Work out the finished part from the listing and answer in its coordinate system (mm). Round coordinates to 2 decimals unless told otherwise and drop trailing zeros. Order: outer loops, then holes, each group sorted by start corner. A loop starts at its lowest first (then second) coordinate and runs counter-clockwise, first axis right, second up. Notation, with made-up numbers: M -34,73.25 L -23,73.25 A11 ccw -23,93.25 Z; hole C 27,89.25 d5. An arc over 180 degrees is marked long. Answer as a JSON object with one key per item and string values. Group by question number.
from build123d import *

# Parameters (mm, degrees)
BOSS_EXTRUDE1_DEPTH = 13.7
SKETCH3_W           = 0.178571672
SKETCH3_H           = 6.380917094
CUT_EXTRUDE1_DEPTH  = 0.2
SKETCH4_R           = 0.85
BOSS_EXTRUDE3_DEPTH = 7.4
SKETCH5_W           = 0.138137893
SKETCH5_H           = 1.329179466
BOSS_EXTRUDE4_DEPTH = 2.8
SKETCH6_R           = 0.20198457
CUT_EXTRUDE2_DEPTH  = 9.6
REDONDEO1_R         = 0.5


with BuildPart() as part:
    # Sketch1 → Boss-Extrude1 (new body)
    with BuildSketch(Plane.XY):
        with BuildLine():
            Line((-3.31662479, -5), (3.31662479, -5))
            ThreePointArc((3.31662479, -5), (6, 0), (3.31662479, 5))
            Line((3.31662479, 5), (-3.31662479, 5))
            ThreePointArc((-3.31662479, 5), (-6, 0), (-3.31662479, -5))
        make_face()
    extrude(amount=BOSS_EXTRUDE1_DEPTH)

    # Sketch3 → Cut-Extrude1 (cut)
    with BuildSketch(Plane(origin=(0, 5, 0), x_dir=(1, 0, 0), z_dir=(0, 1, 0))):
        with Locations((-2.495957535, -5.684471075)):
            Rectangle(SKETCH3_W, SKETCH3_H)
        with Locations((2.495957535, -5.684471075)):
            Rectangle(SKETCH3_W, SKETCH3_H)
    extrude(amount=-CUT_EXTRUDE1_DEPTH, mode=Mode.SUBTRACT)

    # Sketch4 → Boss-Extrude3 (add)
    with BuildSketch(Plane(origin=(0, 0, 0), x_dir=(-1, 0, 0), z_dir=(0, 0, -1))):
        with Locations(Location((0, 0, 0), (0, 0, 180))):
            Circle(SKETCH4_R)
    extrude(amount=BOSS_EXTRUDE3_DEPTH)

    # Sketch5 → Boss-Extrude4 (add)
    with BuildSketch(Plane(origin=(0, 0, 0), x_dir=(-1, 0, 0), z_dir=(0, 0, -1))):
        with Locations((-4.217525365, 0)):
            Rectangle(SKETCH5_W, SKETCH5_H)
        with Locations((4.217525365, 0)):
            Rectangle(SKETCH5_W, SKETCH5_H)
    extrude(amount=BOSS_EXTRUDE4_DEPTH)

    # Sketch6 → Cut-Extrude2 (cut)
    with BuildSketch(Plane.ZY.offset(4.286594311)):
        with Locations((-2.171650698, 0)):
            Circle(SKETCH6_R)
    extrude(amount=-CUT_EXTRUDE2_DEPTH, mode=Mode.SUBTRACT)

    # Redondeo1
    redondeo1_edges = [part.edges().sort_by_distance(p)[0] for p in [
        (-0.85, 0, -7.4),
    ]]
    fillet(redondeo1_edges, radius=REDONDEO1_R)


solid = part.part
Item 1: Find section C-C (x = -2). Give the vertices of the cut face in (y, z).
Item 2: Consider L1, parallel to Z at x = 0.3, y = 0; L2, parallel to Z at x = 4, y = 2.5; L3, parallel to Y at x = 5, z = 11.25. Determine where each line is inside the solid, lowest interval first.
Item 3: Each of these flat-tipped pins is pushed along its axis until it touches: pin 1 (3 mm diameter, centred on x = 2, y = -2, fed in from -Z); pin 2 (1.5 mm diameter, centred on y = 0.5, z = -2, fed in from -X); pin 3 (5 mm diameter, centred on x = 3.5, y = 2.5, fed in from -Z). Where does it stop, or does it pass through?
Item 4: The mould has two halves that part along X. Classify faces 1 (the flat face through (0, 5, 7)), 2 (the cylindrical face through (-0.18, 0.83, -3.4)), 3 (the cylindrical face through (6, 0, 7)): +X half, -X half, draft (parallel to the pull), parting line (faces both ways), or undercut.
Item 5: Find section B-B (y = -2.25). Give the vertices of the cut face in (x, z).
Item 6: Find section A-A (z = 7). Give the vertices of the cut face in (x, y), and give its area (3 significant figures).
Responses:
{
 "1": {"outline": "M -5,0 L 5,0 L 5,13.7 L -5,13.7 Z"},
 "2": {"L1": "z = -7.4 to -2.37, -1.97 to 13.7", "L2": "z = 0 to 13.7", "L3": "y = -3.32 to 3.32"},
 "3": {"pin 1": "stops at z = 0", "pin 2": "stops at x = -4.29", "pin 3": "stops at z = -2.8"},
 "4": {"face 1": "draft", "face 2": "undercut", "face 3": "+X half"},
 "5": {"outline": "M -5.56,0 L 5.56,0 L 5.56,13.7 L -5.56,13.7 Z"},
 "6": {"outline": "M -3.32,-5 L 3.32,-5 A6 ccw 3.32,5 L 2.59,5 L 2.59,4.8 L 2.41,4.8 L 2.41,5 L -2.41,5 L -2.41,4.8 L -2.59,4.8 L -2.59,5 L -3.32,5 A6 ccw Z", "area": "104 mm^2"}
}
